The listing builds one solid part. Answer for the finished solid, in the listing's coordinates (mm). A direction names the side the tool comes from. Coordinates: 2 decimals unless noted, no trailing zeros. Order: outer loops, then holes, each group sorted by start corner. A loop starts at its lowest first (then second) coordinate and runs counter-clockwise, first axis right, second up. Notation, with made-up numbers: (-15, -14) -> (29, -14) arc R17 cw to (29, 5) -> close; hole circle Ø8 at (-0.75, 46). An arc over 180 degrees is marked (long way). Return JSON: item names as keys, results as strings.
from build123d import *

# Parameters (mm, degrees)
SKETCH1_W           = 185
SKETCH1_H           = 60
BOSS_EXTRUDE1_DEPTH = 3
SKETCH2_R           = 1.5
CUT_EXTRUDE1_DEPTH  = 3
CUT_EXTRUDE2_DEPTH  = 10


with BuildPart() as part:
    # Sketch1 → Boss-Extrude1 (new body)
    with BuildSketch(Plane(origin=(0, 0, 0), x_dir=(1, 0, 0), z_dir=(0, 1, 0))):
        with Locations((-80.280821918, -28.849315068)):
            Rectangle(SKETCH1_W, SKETCH1_H)
    extrude(amount=BOSS_EXTRUDE1_DEPTH)

    # Sketch2 → Cut-Extrude1 (cut)
    with BuildSketch(Plane(origin=(0, 3, 0), x_dir=(1, 0, 0), z_dir=(0, 1, 0))):
        with Locations((-163.653280502, -7.099315068)):
            Circle(SKETCH2_R)
        with Locations((-163.653280502, -50.599315068)):
            Circle(SKETCH2_R)
        with Locations((-28.153280502, -50.599315068)):
            Circle(SKETCH2_R)
        with Locations((-28.153280502, -7.099315068)):
            Circle(SKETCH2_R)
        with Locations((-132.986057559, -7.099315068)):
            Circle(SKETCH2_R)
        with Locations((-132.986057559, -50.599315068)):
            Circle(SKETCH2_R)
        with Locations((2.513942441, -50.599315068)):
            Circle(SKETCH2_R)
        with Locations((2.513942441, -7.099315068)):
            Circle(SKETCH2_R)
        with BuildLine():
            Line((-139.976197673, -12.515770436), (-16.64325173, -12.515770436))
            ThreePointArc((-16.64325173, -12.515770436), (-0.309707097, -28.849315068), (-16.64325173, -45.182859701))
            Line((-16.64325173, -45.182859701), (-139.976197673, -45.182859701))
            ThreePointArc((-139.976197673, -45.182859701), (-156.309742305, -28.849315068), (-139.976197673, -12.515770436))
        make_face()
    extrude(amount=-CUT_EXTRUDE1_DEPTH, mode=Mode.SUBTRACT)

    # Mirror1: part across plane


with BuildPart() as part_1:
    add(part.part)
    add(part.part.mirror(Plane(origin=(-172.780821918, 3, 58.849315068), x_dir=(1, 0, 0), z_dir=(0, 0, -1))))

    # Sketch3 → Cut-Extrude2 (cut)
    with BuildSketch(Plane(origin=(0, 3, 0), x_dir=(1, 0, 0), z_dir=(0, 1, 0))):
        with BuildLine():
            Line((-103.404990518, -51.173645659), (-59.281035157, -51.173645659))
            ThreePointArc((-59.281035157, -51.173645659), (-51.253781089, -59.200899728), (-59.281035157, -67.228153796))
            Line((-59.281035157, -67.228153796), (-103.404990518, -67.228153796))
            ThreePointArc((-103.404990518, -67.228153796), (-111.432244586, -59.200899728), (-103.404990518, -51.173645659))
        make_face()
    extrude(amount=-CUT_EXTRUDE2_DEPTH, mode=Mode.SUBTRACT)


solid = part_1.part
1. The part is cut by section D-D on y = 1.75. Give the number of separate pieces and of enclosed holes in the cut face, and give its area (3 significant figures).
Answer block:
{"separate pieces": "1", "enclosed holes": "19", "area": "11,400 mm2"}
2. Determine the mould class of faces 1 (the face through (-0.314, 1.521, 89.208)), 2 (the face through (-111.43, 1.52, 59.38)), 3 (the face through (-82, 3, 46)) for opening direction Z: pulls with the +Z half, pulls with the -Z half, needs draft (parallel to the pull), parting line crosses it, or undercut.
Answer block:
{"face 1": "undercut", "face 2": "undercut", "face 3": "needs draft"}
3. The part is cut by section C-C on x = -79. Give the vertices of the cut face in (y, z), and give its area (3 significant figures).
Answer block:
{"outline": "(0, -1.15) -> (3, -1.15) -> (3, 12.52) -> (0, 12.52) -> close; (0, 45.18) -> (3, 45.18) -> (3, 51.17) -> (0, 51.17) -> close; (0, 67.23) -> (3, 67.23) -> (3, 72.52) -> (0, 72.52) -> close; (0, 105.18) -> (3, 105.18) -> (3, 118.85) -> (0, 118.85) -> close", "area": "116 mm2"}
4. The part is cut by section B-B on z = 77.5. Give the vertices of the cut face in (x, y).
Answer block:
{"outline": "(-172.78, 0) -> (-151.72, 0) -> (-151.72, 3) -> (-172.78, 3) -> close; (-4.9, 0) -> (12.22, 0) -> (12.22, 3) -> (-4.9, 3) -> close"}
5. Consider line 1 (Z direction, x = -35.5, y = 0.35); line 2 (Z direction, x = -80, y = 1.7); line 3 (X direction, y = 1.55, z = 28.5). Determine where each line is inside the solid, lowest interval first. Write a range as from..to.
Answer block:
{"line 1": "z = -1.15..12.52, 45.18..72.52, 105.18..118.85", "line 2": "z = -1.15..12.52, 45.18..51.17, 67.23..72.52, 105.18..118.85", "line 3": "x = -172.78..-156.31, -0.31..12.22"}
6. This flat-tipped pin is pushed along its axis until it touches: pin 1 Ø1.8 at (x, z) = (-28.15, 50.6) entering from -Y. Where does it stop, or does it pass through?
Answer block:
{"pin 1": "passes through"}
7. For faces 4 (the face through (-82, 0, 46)), 5 (the face through (-0.314, 1.521, 28.49)), determine the directions among +Z, -Z, +X, -X, +Y, -Y from which every point of the face is accessible in a straight line to the end or side of a thin tool.
Answer block:
{"face 4": "+Z, -Z, +X, -X, -Y", "face 5": "+Y, -Y"}
8. The part is cut by section A-A on x = -151. Give the vertices of the cut face in (y, z).
Answer block:
{"outline": "(0, -1.15) -> (3, -1.15) -> (3, 16.8) -> (0, 16.8) -> close; (0, 40.9) -> (3, 40.9) -> (3, 76.8) -> (0, 76.8) -> close; (0, 100.9) -> (3, 100.9) -> (3, 118.85) -> (0, 118.85) -> close"}
